```python
from build123d import *

# Parameters (mm, degrees)
SKETCH2_R             = 3.9751
BOSS_EXTRUDE1_DEPTH   = 17.2
M3X0_5_TAPPED_HOLE1_D = 2.5
SKETCH5_R             = 3.9751
SKETCH5_R_2           = 3.5
CUT_EXTRUDE1_DEPTH    = 4.675
SKETCH6_R             = 3.5
SKETCH6_R_2           = 2
CUT_EXTRUDE2_DEPTH    = 1
SKETCH7_R             = 3.9751
SKETCH7_R_2           = 3.5
CUT_EXTRUDE3_DEPTH    = 10.675
SKETCH8_R             = 3.5
SKETCH8_R_2           = 2
CUT_EXTRUDE4_DEPTH    = 1


with BuildPart() as part:
    # Sketch2 → Boss-Extrude1 (new body, symmetric)
    with BuildSketch(Plane(origin=(0, 0, 0), x_dir=(1, 0, 0), z_dir=(0, 1, 0))):
        Circle(SKETCH2_R)
    extrude(amount=BOSS_EXTRUDE1_DEPTH, both=True)

    # M3x0.5 Tapped Hole1 (through all)
    with Locations(Plane(origin=(0, 17.2, 0), x_dir=(1, 0, 0), z_dir=(0, 1, 0))):
        with Locations((0, 0)):
            Hole(M3X0_5_TAPPED_HOLE1_D / 2)

    # Sketch5 → Cut-Extrude1 (cut)
    with BuildSketch(Plane(origin=(0, 17.2, 0), x_dir=(1, 0, 0), z_dir=(0, 1, 0))):
        Circle(SKETCH5_R)
        Circle(SKETCH5_R_2, mode=Mode.SUBTRACT)
    extrude(amount=-CUT_EXTRUDE1_DEPTH, mode=Mode.SUBTRACT)

    # Sketch6 → Cut-Extrude2 (cut)
    with BuildSketch(Plane(origin=(0, 17.2, 0), x_dir=(1, 0, 0), z_dir=(0, 1, 0))):
        Circle(SKETCH6_R)
        Circle(SKETCH6_R_2, mode=Mode.SUBTRACT)
    extrude(amount=-CUT_EXTRUDE2_DEPTH, mode=Mode.SUBTRACT)

    # Sketch7 → Cut-Extrude3 (cut)
    with BuildSketch(Plane.XZ.offset(17.2)):
        Circle(SKETCH7_R)
        Circle(SKETCH7_R_2, mode=Mode.SUBTRACT)
    extrude(amount=-CUT_EXTRUDE3_DEPTH, mode=Mode.SUBTRACT)

    # Sketch8 → Cut-Extrude4 (cut)
    with BuildSketch(Plane.XZ.offset(17.2)):
        Circle(SKETCH8_R)
        Circle(SKETCH8_R_2, mode=Mode.SUBTRACT)
    extrude(amount=-CUT_EXTRUDE4_DEPTH, mode=Mode.SUBTRACT)


solid = part.part
```
Geometry: final body of the model. Coordinates: model frame, mm. A direction names the side the tool comes from. Round coordinates to 2 decimals unless told otherwise and drop trailing zeros. Order: outer loops, then holes, each group sorted by start corner. A loop starts at its lowest first (then second) coordinate and runs counter-clockwise, first axis right, second up. Notation, with made-up numbers: (72.25, -24) -> (98.25, -24) arc R20 ccw to (98.25, 6) -> close; hole circle Ø11 at (25, 72.5). An arc over 180 degrees is marked (long way). Use CSV: the item, a comma, the result in double quotes. Start each with the question number.
1) Section D-D (x = -2.75). Return the cut outline in (y, z) (3 decimals).
2) Section C-C (y = 1). Return the cut outline in (x, z), and give its area (3 significant figures).
3) First-contact query: pin 1 Ø2 at (x, z) = (0, 0) entering from +Y; pin 2 Ø4 at (x, z) = (3, -3) entering from +Y. Flat tips, straight axial feed; report the tip coordinate or a pass-through.
4) Set-up query: faces 1 (the face through (3.233, 14.388, 1.341)), 2 (the face through (3.233, -11.43, -1.341)), 3 (the face through (1, -17.2, -1)). Return all of +Z, -Z, +X, -X, +Y, -Y with unobstructed straight access to the full face (end or side cutting, diameter ignored); none if empty.
5) Section A-A (x = 0). Return the cut outline in (y, z) (3 decimals).
6) Material intervals for line 1 along Z through (x, y) = (0, 6); line 2 along Z through (x, y) = (0, -7.5); line 3 along Y through (x, z) = (1.75, -2), sorted ascending. Write a range as from..to.
7) Section B-B (z = 0). Return the cut outline in (x, y) (3 decimals).
8) Draft query along X for faces 4 (the face through (2, -16.2, -2)), 5 (the face through (0.27, -0.24, 1.22)), 6 (the face through (0, -17, -2)). Return one class per face: +X half, -X half, draft (parallel to the pull), parting line (faces both ways), or undercut.
Returned:
1,outline,"(-16.2, -2.165) -> (-6.525, -2.165) -> (-6.525, -2.87) -> (12.525, -2.87) -> (12.525, -2.165) -> (16.2, -2.165) -> (16.2, 2.165) -> (12.525, 2.165) -> (12.525, 2.87) -> (-6.525, 2.87) -> (-6.525, 2.165) -> (-16.2, 2.165) -> close"
2,outline,"circle Ø7.95 at (0, 0); hole circle Ø2.5 at (0, 0)"
2,area,"44.7 mm²"
3,pin 1,"passes through"
3,pin 2,"stops at y = 16.2"
4,face 1,"+Y"
4,face 2,"-Y"
4,face 3,"+Z, -Z, +X, -X, -Y"
5,outline,"(-17.2, -2) -> (-16.2, -2) -> (-16.2, -3.5) -> (-6.525, -3.5) -> (-6.525, -3.975) -> (12.525, -3.975) -> (12.525, -3.5) -> (16.2, -3.5) -> (16.2, -2) -> (17.2, -2) -> (17.2, -1.25) -> (-17.2, -1.25) -> close; (-17.2, 1.25) -> (17.2, 1.25) -> (17.2, 2) -> (16.2, 2) -> (16.2, 3.5) -> (12.525, 3.5) -> (12.525, 3.975) -> (-6.525, 3.975) -> (-6.525, 3.5) -> (-16.2, 3.5) -> (-16.2, 2) -> (-17.2, 2) -> close"
6,line 1,"z = -3.98..-1.25, 1.25..3.98"
6,line 2,"z = -3.5..-1.25, 1.25..3.5"
6,line 3,"y = -16.2..16.2"
7,outline,"(-3.975, -6.525) -> (-3.5, -6.525) -> (-3.5, -16.2) -> (-2, -16.2) -> (-2, -17.2) -> (-1.25, -17.2) -> (-1.25, 17.2) -> (-2, 17.2) -> (-2, 16.2) -> (-3.5, 16.2) -> (-3.5, 12.525) -> (-3.975, 12.525) -> close; (1.25, -17.2) -> (2, -17.2) -> (2, -16.2) -> (3.5, -16.2) -> (3.5, -6.525) -> (3.975, -6.525) -> (3.975, 12.525) -> (3.5, 12.525) -> (3.5, 16.2) -> (2, 16.2) -> (2, 17.2) -> (1.25, 17.2) -> close"
8,face 4,"draft"
8,face 5,"undercut"
8,face 6,"parting line"
